Source: CAD feature listing. Evaluate the final solid. Frame: model axes, mm. A direction names the side the tool comes from. Give positions to 0.01 mm unless a question says otherwise; leave off trailing zeros. Order: outer loops, then holes, each group sorted by start corner. A loop starts at its lowest first (then second) coordinate and runs counter-clockwise, first axis right, second up. Notation, with made-up numbers: M 50,40 L 107,40 A21 ccw 107,49 Z; hole C 79.5,80 d9. An arc over 180 degrees is marked long. Answer in a Markdown table with one row per item. Add a question column.
(1) Material intervals for line 1 along X through (y, z) = (-15.5, 10); line 2 along Y through (x, z) = (30, 2); line 3 along X through (y, z) = (-38, 2), sorted ascending.
(2) Mould query, pull axis X, two halves, no side actions, for faces 1 (the face through (28.85, -18, 8)), 2 (the face through (35.419, -76.094, 4.388)), 3 (the face through (37, 10.8, 4)). Classes: pulls with the +X half, pulls with the -X half, needs draft (parallel to the pull), parting line crosses it, or undercut.
(3) Pin query (flat end, axial travel): P1, Ø1.9, axis at x = -31.5, y = -72.5, coming from the -Z side; P2, Ø1.6, axis at x = 36.5, z = 3, coming from the +Y side; P3, Ø4.5, axis at y = -74, z = 9.5, coming from the +X side. Return the tip coordinate at first contact, or that it passes through.
(4) Section query A-A, the plane y = -25. Return loops of the section in (x, z), plus the area to 3 significant figures.
(5) Section query B-B, the plane x = -11.5. Return loops of the section in (y, z).
(6) Set-up query: faces 4 (the face through (22, -18.664, 14)), 5 (the face through (34, 12.5, 8)), 6 (the face through (-25.8, 21, 2)), 7 (the face through (22, -47, -2)). Return all of +Z, -Z, +X, -X, +Y, -Y with unobstructed straight access to the full face (end or side cutting, diameter ignored); none if empty.
from build123d import *

# Parameters (mm, degrees)
SKETCH_W        = 75.4
SKETCH_H        = 100
PAD_DEPTH       = 16.6
SKETCH005_W     = 71.4
SKETCH005_H     = 96
POCKET_DEPTH    = 14.6
SKETCH006_W     = 21.6
SKETCH006_H     = 12
POCKET001_DEPTH = 2
SKETCH007_W     = 21.6
SKETCH007_H     = 12
POCKET002_DEPTH = 2
SKETCH008_W     = 7.6
SKETCH008_H     = 8.2
POCKET003_DEPTH = 2
SKETCH009_R     = 1.85
POCKET004_DEPTH = 2
SKETCH010_R     = 3.9
POCKET005_DEPTH = 2
POCKET005_TAPER = 45
SKETCH011_W     = 15
SKETCH011_H     = 2
PAD005_DEPTH    = 14.6
SKETCH012_R     = 0.9
PAD006_DEPTH    = 8.6
SKETCH013_R     = 0.9
PAD007_DEPTH    = 10.4
FILLET_R        = 2
FILLET001_R     = 4
FILLET002_R     = 1
FILLET003_R     = 6
FILLET004_R     = 8
FILLET005_R     = 4


with BuildPart() as part:
    # Sketch → Pad (new body)
    with BuildSketch(Plane.XY):
        with Locations((0, -28.5)):
            Rectangle(SKETCH_W, SKETCH_H)
    extrude(amount=PAD_DEPTH)

    # Sketch005 (on Face5 of Pad) → Pocket (cut)
    with BuildSketch(Plane(origin=(0, 0, 0), x_dir=(1, 0, 0), z_dir=(0, 0, -1))):
        with Locations((0, 28.5)):
            Rectangle(SKETCH005_W, SKETCH005_H)
    extrude(amount=-POCKET_DEPTH, mode=Mode.SUBTRACT)

    # Sketch006 (on Face3 of Pocket) → Pocket001 (cut)
    with BuildSketch(Plane.YZ.offset(37.7)):
        with Locations((0, 6)):
            Rectangle(SKETCH006_W, SKETCH006_H)
    extrude(amount=-POCKET001_DEPTH, mode=Mode.SUBTRACT)

    # Sketch007 (on Face2 of Pocket) → Pocket002 (cut)
    with BuildSketch(Plane(origin=(-37.7, 0, 0), x_dir=(0, -1, 0), z_dir=(-1, 0, 0))):
        with Locations((0, 6)):
            Rectangle(SKETCH007_W, SKETCH007_H)
    extrude(amount=-POCKET002_DEPTH, mode=Mode.SUBTRACT)

    # Sketch008 (on Face1 of Pocket) → Pocket003 (cut)
    with BuildSketch(Plane(origin=(0, 21.5, 0), x_dir=(-1, 0, 0), z_dir=(0, 1, 0))):
        with Locations((22, 4.1)):
            Rectangle(SKETCH008_W, SKETCH008_H)
    extrude(amount=-POCKET003_DEPTH, mode=Mode.SUBTRACT)

    # Sketch009 (on Face5 of Pocket) → Pocket004 (cut)
    with BuildSketch(Plane.XY.offset(16.6)):
        with Locations((21.601854, -2.031842)):
            Circle(SKETCH009_R)
        with Locations((21.597205, 5.352823)):
            Circle(SKETCH009_R)
        with BuildLine():
            Line((15.825713, -15.337742), (15.825713, -16.321696))
            ThreePointArc((15.825713, -16.321696), (16.397859, -17.902616), (17.897046, -18.663599))
            Line((17.897046, -18.663599), (25.282393, -18.663599))
            ThreePointArc((25.282393, -18.663599), (26.185781, -18.272491), (26.544973, -17.355945))
            Line((26.544973, -14.219638), (26.544973, -17.355945))
            ThreePointArc((26.544973, -14.219638), (26.159832, -13.349897), (25.274241, -13.00275))
            Line((17.921865, -13.00275), (25.274241, -13.00275))
            ThreePointArc((17.921865, -13.00275), (16.411472, -13.755218), (15.825713, -15.337742))
        make_face()
    extrude(amount=-POCKET004_DEPTH, mode=Mode.SUBTRACT)

    # Sketch010 (on Face5 of Pocket) → Pocket005 (cut)
    with BuildSketch(Plane.XY.offset(16.6)):
        with Locations((-17.145816, -1.900756)):
            Circle(SKETCH010_R)
    extrude(amount=-POCKET005_DEPTH, taper=POCKET005_TAPER, mode=Mode.SUBTRACT)

    # Sketch011 (on Face11 of Pocket) → Pad005 (join)
    with BuildSketch(Plane(origin=(0, 0, 14.6), x_dir=(1, 0, 0), z_dir=(0, 0, -1))):
        with Locations((-28.2, 47.5)):
            Rectangle(SKETCH011_W, SKETCH011_H)
        with Locations((-28.2, 20.5)):
            Rectangle(SKETCH011_W, SKETCH011_H)
        with Locations((28.2, 47.5)):
            Rectangle(SKETCH011_W, SKETCH011_H)
        with Locations((28.2, 20.5)):
            Rectangle(SKETCH011_W, SKETCH011_H)
    extrude(amount=PAD005_DEPTH)

    # Sketch012 (on Face11 of Pocket) → Pad006 (join)
    with BuildSketch(Plane(origin=(0, 0, 14.6), x_dir=(1, 0, 0), z_dir=(0, 0, -1))):
        with BuildLine():
            Line((-35.7, -12.5), (-31.85, -12.5))
            ThreePointArc((-28.85, -15.5), (-29.72868, -13.37868), (-31.85, -12.5))
            Line((-28.85, -19.5), (-28.85, -15.5))
            Line((-28.85, -19.5), (-35.7, -19.5))
            Line((-35.7, -12.5), (-35.7, -19.5))
        make_face()
        with Locations((-31.85, -15.5)):
            Circle(SKETCH012_R, mode=Mode.SUBTRACT)
        with BuildLine():
            Line((28.85, -19.5), (28.85, -15.5))
            ThreePointArc((31.85, -12.5), (29.72868, -13.37868), (28.85, -15.5))
            Line((35.7, -12.5), (31.85, -12.5))
            Line((35.7, -12.5), (35.7, -19.5))
            Line((28.85, -19.5), (35.7, -19.5))
        make_face()
        with Locations((31.85, -15.5)):
            Circle(SKETCH012_R, mode=Mode.SUBTRACT)
        with BuildLine():
            Line((-35.7, 12.5), (-35.7, 19.5))
            Line((-35.7, 19.5), (-28.85, 19.5))
            Line((-28.85, 19.5), (-28.85, 15.5))
            ThreePointArc((-31.85, 12.5), (-29.72868, 13.37868), (-28.85, 15.5))
            Line((-35.7, 12.5), (-31.85, 12.5))
        make_face()
        with Locations((-31.85, 15.5)):
            Circle(SKETCH012_R, mode=Mode.SUBTRACT)
        with BuildLine():
            Line((31.85, 12.5), (35.7, 12.5))
            Line((35.7, 12.5), (35.7, 19.5))
            Line((35.7, 19.5), (28.85, 19.5))
            Line((28.85, 19.5), (28.85, 15.5))
            ThreePointArc((28.85, 15.5), (29.72868, 13.37868), (31.85, 12.5))
        make_face()
        with Locations((31.85, 15.5)):
            Circle(SKETCH012_R, mode=Mode.SUBTRACT)
    extrude(amount=PAD006_DEPTH)

    # Sketch013 (on Face11 of Pocket) → Pad007 (join)
    with BuildSketch(Plane(origin=(0, 0, 14.6), x_dir=(1, 0, 0), z_dir=(0, 0, -1))):
        with BuildLine():
            Line((-35.7, 76.5), (-29.35, 76.5))
            Line((-29.35, 76.5), (-29.35, 72.5))
            ThreePointArc((-31.85, 70), (-30.082233, 70.732233), (-29.35, 72.5))
            Line((-35.7, 70), (-31.85, 70))
            Line((-35.7, 76.5), (-35.7, 70))
        make_face()
        with Locations((-31.85, 72.5)):
            Circle(SKETCH013_R, mode=Mode.SUBTRACT)
        with BuildLine():
            Line((35.7, 76.5), (35.7, 70))
            Line((35.7, 70), (31.85, 70))
            ThreePointArc((29.35, 72.5), (30.082233, 70.732233), (31.85, 70))
            Line((29.35, 76.5), (29.35, 72.5))
            Line((35.7, 76.5), (29.35, 76.5))
        make_face()
        with Locations((31.85, 72.5)):
            Circle(SKETCH013_R, mode=Mode.SUBTRACT)
    extrude(amount=PAD007_DEPTH)

    # Fillet
    fillet_edges = [part.edges().sort_by_distance(p)[0] for p in [
        (-35.7, 0, 14.6),
        (-35.7, -34, 14.6),
        (-35.7, -59.25, 14.6),
        (35.7, -59.25, 14.6),
        (35.7, -34, 14.6),
        (35.7, 0, 14.6),
    ]]
    fillet(fillet_edges, radius=FILLET_R)

    # Fillet001
    fillet001_edges = [part.edges().sort_by_distance(p)[0] for p in [
        (0, 19.5, 14.6),
        (0, -76.5, 14.6),
    ]]
    fillet(fillet001_edges, radius=FILLET001_R)

    # Fillet002
    fillet002_edges = [part.edges().sort_by_distance(p)[0] for p in [
        (-35.7, 19.5, 3),
        (35.7, 19.5, 3),
    ]]
    fillet(fillet002_edges, radius=FILLET002_R)

    # Fillet003
    fillet003_edges = [part.edges().sort_by_distance(p)[0] for p in [
        (-35.7, -76.5, 2.1),
        (35.7, -76.5, 2.1),
    ]]
    fillet(fillet003_edges, radius=FILLET003_R)

    # Fillet004
    fillet004_edges = [part.edges().sort_by_distance(p)[0] for p in [
        (37.7, -78.5, 8.3),
        (0, -78.5, 16.6),
        (-37.7, -78.5, 8.3),
        (0, 21.5, 16.6),
    ]]
    fillet(fillet004_edges, radius=FILLET004_R)

    # Fillet005
    fillet005_edges = [part.edges().sort_by_distance(p)[0] for p in [
        (37.7, -28.5, 16.6),
        (37.7, 21.5, 4.3),
        (37.7, 19.156854, 14.256854),
        (-37.7, 21.5, 4.3),
        (-37.7, 19.156854, 14.256854),
        (-37.7, -28.5, 16.6),
        (-34.868391, -76.606368, 13.768391),
        (34.868391, -76.606368, 13.768391),
    ]]
    fillet(fillet005_edges, radius=FILLET005_R)


with BuildPart() as part_1:
    # Body placement: moved
    add(part.part.moved(Location((0, 0, -2))))


solid = part_1.part
Values follow:
| question | item | result |
|---|---|---|
| 1 | line 1 | x = -37.7 to -32.75, -30.95 to -28.85, 28.85 to 30.95, 32.75 to 37.7 |
| 1 | line 2 | y = -78.49 to -76.49, -48.5 to -46.5, -21.5 to -19.5, 19.5 to 21.5 |
| 1 | line 3 | x = -37.7 to -35.7, 35.7 to 37.7 |
| 2 | face 1 | undercut |
| 2 | face 2 | pulls with the +X half |
| 2 | face 3 | needs draft |
| 3 | P1 | stops at z = 2.2 |
| 3 | P2 | stops at y = 20.96 |
| 3 | P3 | stops at x = 37.6 |
| 4 | outline | M -37.7,-2 L -35.7,-2 L -35.7,10.6 A2 cw -33.7,12.6 L 33.7,12.6 A2 cw 35.7,10.6 L 35.7,-2 L 37.7,-2 L 37.7,10.6 A4 ccw 33.7,14.6 L -33.7,14.6 A4 ccw -37.7,10.6 Z |
| 4 | area | 204 mm² |
| 5 | outline | M -78.5,-2 L -76.5,-2 L -76.5,8.6 A4 cw -72.5,12.6 L 15.5,12.6 A4 cw 19.5,8.6 L 19.5,-2 L 21.5,-2 L 21.5,6.6 A8 ccw 13.5,14.6 L -70.5,14.6 A8 ccw -78.5,6.6 Z |
| 6 | face 4 | +Z, -Z |
| 6 | face 5 | -Z |
| 6 | face 6 | -Z, +Y |
| 6 | face 7 | -Z, +X, -X, +Y, -Y |
